```python
from build123d import *

# Parameters (mm, degrees)
F0_W     = 108.7121069431
F0_H     = 140.9654691815
F0_W_2   = 95.1121076941
F0_H_2   = 127.3654699326
F1_DEPTH = 88.9
F2_W     = 108.7121069431
F2_H     = 140.9654691815
F3_DEPTH = 3.8
F4_W     = 101.9121073186
F4_H     = 134.165469557
F5_DEPTH = 88.9
F6_W     = 35.625605844
F6_H     = 5.0125271082
F7_DEPTH = 82.4


with BuildPart() as f1:
    # F0 (on Top) → F1 (new body)
    with BuildSketch(Plane.XY):
        Rectangle(F0_W, F0_H)
        Rectangle(F0_W_2, F0_H_2, mode=Mode.SUBTRACT)
    extrude(amount=F1_DEPTH)

    # F2 (on face) → F3 (join)
    with BuildSketch(Plane(origin=(0, 0, 0), x_dir=(1, 0, 0), z_dir=(0, 0, -1))):
        Rectangle(F2_W, F2_H)
    extrude(amount=F3_DEPTH)

    # F4 (on face) → F5 (cut, through all)
    with BuildSketch(Plane.XY.offset(88.9)):
        with Locations((3.3999998122, -3.3999998122)):
            Rectangle(F4_W, F4_H)
    extrude(amount=-F5_DEPTH, mode=Mode.SUBTRACT)

    # F6 (on face) → F7 (join)
    with BuildSketch(Plane.XZ.offset(-63.6827349663)):
        with Locations((-29.7432509251, 64.6251067519)):
            Rectangle(F6_W, F6_H)
    extrude(amount=F7_DEPTH)


solid = f1.part
```
Here's how the part is built. I have some questions about the finished solid (model axes, mm). A direction names the side the tool comes from. Round coordinates to 2 decimals unless told otherwise and drop trailing zeros. Loops run counter-clockwise (first coordinate to the right, second up) from the corner with the lowest first, then second, coordinate; pieces in that order, holes last.
1. Will these pins go through, and if not, where does the flat tip stop? pin 1 (1.5 mm diameter, centred on y = 31, z = 64.5, fed in from +X); pin 2 (6 mm diameter, centred on y = -23, z = 73.5, fed in from +X); pin 3 (2.5 mm diameter, centred on x = -25, z = 64.5, fed in from -Y).
Answers:
pin 1: stops at x = -11.93
pin 2: stops at x = -47.56
pin 3: stops at y = -18.72
2. If I drill on probe 1 along Z at (x, y) = (-37.5, 9); probe 2 along Y at (x, z) = (-26, 47); probe 3 along Z at (x, y) = (22, 56.5), over which ranges is the centre line in solid material (lowest first)?
Answers:
probe 1: z = -3.8 to 0, 62.12 to 67.13
probe 2: y = 63.68 to 70.48
probe 3: z = -3.8 to 0
3. Suppose I cut it at D-D, the plane x = 28. Please give me the cut outline in (y, z).
Answers:
outline: (-70.48, -3.8) - (70.48, -3.8) - (70.48, 88.9) - (63.68, 88.9) - (63.68, 0) - (-70.48, 0) - close
4. Thinking about a two-plate mould opening in Z: for faces 1 (the face through (3, 63.683, 45)), 2 (the face through (-11.93, 23, 65)), 3 (the face through (-1, -1, -3.8)), which applies, released by +Z, released by -Z, zero draft, split by the parting line, or undercut?
Answers:
face 1: undercut
face 2: zero draft
face 3: released by -Z
5. Suppose I cut it at C-C, the plane z = 36. Please give me the cut outline in (x, y).
Answers:
outline: (-54.36, -70.48) - (-47.56, -70.48) - (-47.56, 63.68) - (54.36, 63.68) - (54.36, 70.48) - (-54.36, 70.48) - close
6. Suppose I cut it at B-B, the plane y = 15. Please give me the cut outline in (x, z).
Answers:
outline: (-54.36, -3.8) - (54.36, -3.8) - (54.36, 0) - (-47.56, 0) - (-47.56, 62.12) - (-11.93, 62.12) - (-11.93, 67.13) - (-47.56, 67.13) - (-47.56, 88.9) - (-54.36, 88.9) - close
7. For faces 4 (the face through (3, -2, 0)), 5 (the face through (54.356, 32, -2)), 6 (the face through (-30, -18.717, 65)), which set-ups out of +Z, -Z, +X, -X, +Y, -Y let a thin tool reach every point of the face, with its end or its side?
Answers:
face 4: +X, -Y
face 5: +Z, -Z, +X, +Y, -Y
face 6: +Z, +X, -Y
8. Suppose I cut it at A-A, the plane x = -40. Please give me the cut outline in (y, z), and give its area (3 significant figures).
Answers:
outline: (-70.48, -3.8) - (70.48, -3.8) - (70.48, 88.9) - (63.68, 88.9) - (63.68, 67.13) - (-18.72, 67.13) - (-18.72, 62.12) - (63.68, 62.12) - (63.68, 0) - (-70.48, 0) - close
area: 1,550 mm2
